Check sheet for the modelled part. Datum: model origin and axes. Units: mm. Face numbers are marked on the shaded views. A direction names the side the tool comes from. Round coordinates to 2 decimals unless told otherwise and drop trailing zeros. Write each loop counter-clockwise with the first axis right and the second up, starting at its lowest first coordinate (ties: lowest second). Pieces come first, ordered by that corner, then holes. Notation, with made-up numbers: (22, 68.25) - (70, 68.25) arc R34 ccw to (70, 103.25) - close; hole circle Ø1 at (54.25, 47.25). An arc over 180 degrees is marked (long way). Answer as a JSON object with one key per item and string values. Group by question number.
Item 1: Thickness scan on line 1 (Y direction, x = 19.05, z = -3.7); line 2 (Z direction, x = 5.5, y = 2.25); line 3 (Y direction, x = 6, z = 4.75). Record the ranges inside material, lowest first.
Item 2: Gauge pin test, flat ends, axial feed: P1, Ø2.5, axis at x = 20, z = 1.5, coming from the +Y side; P2, Ø4.5, axis at x = 19.05, y = 14.525, coming from the +Z side; P3, Ø4, axis at y = 7, z = -2.5, coming from the -X side; P4, Ø1.8, axis at x = 6.35, y = 8.175, coming from the +Z side. Record the tip position at first contact, or that the pin passes through.
Item 3: Sectioned sample at A-A on y = -2. Record the boundary of the cut face in (x, z).
Item 4: Release check for a two-part mould opening along Y. For the marked faces 4, 5, 6 and 7 record: pulls with the +Y half, pulls with the -Y half, needs draft (parallel to the pull), parting line crosses it, or undercut.
Item 5: Sectioned sample at D-D on z = -3.5. Record the boundary of the cut face in (x, y) (3 decimals).
Item 6: Sectioned sample at B-B on x = 25. Record the boundary of the cut face in (y, z), plus the area to 3 significant figures.
Item 7: Sectioned sample at C-C on x = 19.05. Record the boundary of the cut face in (y, z), plus the area to 3 significant figures.
Item 8: Set-up check for the marked faces 1, 2 and 3: record each of +Z, -Z, +X, -X, +Y, -Y from which the full face is reachable in a straight line by a thin tool's end or side.
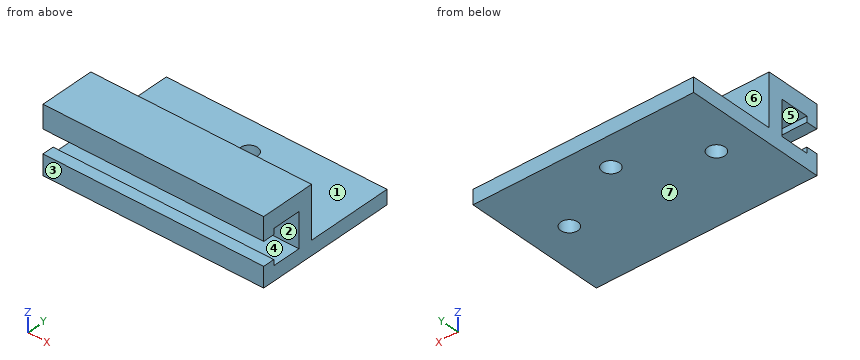
```python
from build123d import *

# Parameters (mm, degrees)
BOSS_EXTRUDE1_DEPTH       = 38.1
F_4_CLEARANCE_HOLE1_D     = 2.9464
F_4_CLEARANCE_HOLE1_DEPTH = 6.35
F_4_CLEARANCE_HOLE1_TIP   = 0.885187864


with BuildPart() as part:
    # Sketch1 → Boss-Extrude1 (new body)
    with BuildSketch(Plane(origin=(0, 0, 0), x_dir=(0, 0, -1), z_dir=(1, 0, 0))):
        Polygon((-6, -4.5), (-2, -4.5), (-2, -2.5), (-3, -2.5), (-3, 2.5), (3, 2.5), (3, -2.5), (2, -2.5), (2, -4.5), (5.5, -4.5), (5.5, 4.583333333), (5.5, 20), (3, 20), (3, 5), (-6, 5), align=None)
    extrude(amount=BOSS_EXTRUDE1_DEPTH)

    # #4 Clearance Hole1
    with Locations(Plane(origin=(0, 0, -5.5), x_dir=(-1, 0, 0), z_dir=(0, 0, -1))):
        with Locations((-19.05, 14.525), (-31.75, 8.175), (-6.35, 8.175)):
            Hole(F_4_CLEARANCE_HOLE1_D / 2, depth=F_4_CLEARANCE_HOLE1_DEPTH)
            with Locations((0, 0, -(F_4_CLEARANCE_HOLE1_DEPTH + F_4_CLEARANCE_HOLE1_TIP / 2))):  # 118° drill point
                Cone(0, F_4_CLEARANCE_HOLE1_D / 2, F_4_CLEARANCE_HOLE1_TIP, mode=Mode.SUBTRACT)


solid = part.part
```
Completed:
{
 "1": {"line 1": "-4.5 to 13.05, 16 to 20", "line 2": "-5.5 to -3, 3 to 6", "line 3": "-4.5 to 5"},
 "2": {"P1": "y = 5", "P2": "z = -3", "P3": "x = 0", "P4": "through"},
 "3": {"outline": "(0, -5.5) - (38.1, -5.5) - (38.1, -3) - (0, -3) - close; (0, 3) - (38.1, 3) - (38.1, 6) - (0, 6) - close"},
 "4": {"face 4": "undercut", "face 5": "undercut", "face 6": "pulls with the +Y half", "face 7": "needs draft"},
 "5": {"outline": "(0, -4.5) - (38.1, -4.5) - (38.1, 20) - (0, 20) - close; hole circle Ø2.946 at (6.35, 8.175); hole circle Ø2.946 at (19.05, 14.525); hole circle Ø2.946 at (31.75, 8.175)"},
 "6": {"outline": "(-4.5, -5.5) - (20, -5.5) - (20, -3) - (5, -3) - (5, 6) - (-4.5, 6) - (-4.5, 2) - (-2.5, 2) - (-2.5, 3) - (2.5, 3) - (2.5, -3) - (-2.5, -3) - (-2.5, -2) - (-4.5, -2) - close", "area": "109 mm²"},
 "7": {"outline": "(-4.5, -5.5) - (13.05, -5.5) - (13.05, -3) - (5, -3) - (5, 6) - (-4.5, 6) - (-4.5, 2) - (-2.5, 2) - (-2.5, 3) - (2.5, 3) - (2.5, -3) - (-2.5, -3) - (-2.5, -2) - (-4.5, -2) - close; (16, -5.5) - (20, -5.5) - (20, -3) - (16, -3) - close", "area": "101 mm²"},
 "8": {"face 1": "+Z, +X, -X, +Y", "face 2": "+X, -X", "face 3": "+Z, -Z, +X, -X, -Y"}
}
